```python
from build123d import *

# Parameters (mm, degrees)
SKETCH1_R           = 12.5
BOSS_EXTRUDE1_DEPTH = 5
BOSS_EXTRUDE1_TAPER = 45
FILLET2_R           = 2.5
SKETCH2_R           = 5
CUT_EXTRUDE1_DEPTH  = 3


with BuildPart() as part:
    # Sketch1 → Boss-Extrude1 (new body)
    with BuildSketch(Plane(origin=(0, 0, 0), x_dir=(1, 0, 0), z_dir=(0, 1, 0))):
        Circle(SKETCH1_R)
    extrude(amount=BOSS_EXTRUDE1_DEPTH, taper=BOSS_EXTRUDE1_TAPER)

    # Fillet2
    fillet2_edges = [part.edges().sort_by_distance(p)[0] for p in [
        (-7.5, 5, 0),
    ]]
    fillet(fillet2_edges, radius=FILLET2_R)

    # Sketch2 → Cut-Extrude1 (cut)
    with BuildSketch(Plane.XZ):
        with Locations(Location((0, 0, 0), (0, 0, 270))):
            Circle(SKETCH2_R)
    extrude(amount=-CUT_EXTRUDE1_DEPTH, mode=Mode.SUBTRACT)


solid = part.part
```
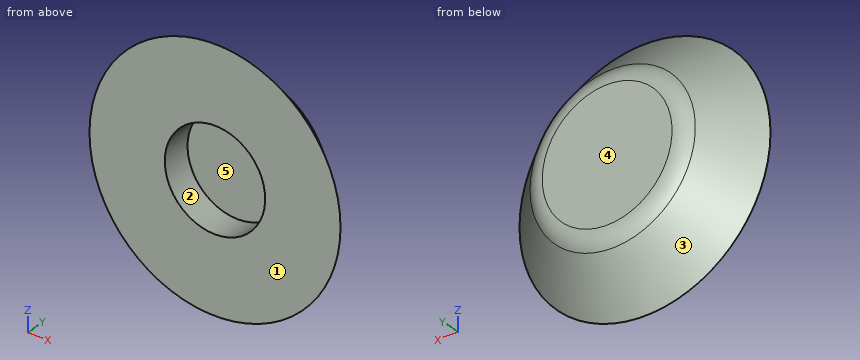
Part model, mm, in its own coordinate system. Face numbers are marked on the shaded views. A direction names the side the tool comes from. Round coordinates to 2 decimals unless told otherwise and drop trailing zeros. Loops run counter-clockwise (first coordinate to the right, second up) from the corner with the lowest first, then second, coordinate; pieces in that order, holes last.
1. Slice it at A-A (y = 1.25). Give the cut face in (x, z), and give its area (3 significant figures).
Solutions:
outline: circle Ø22.5 at (0, 0); hole circle Ø10 at (0, 0)
area: 319 mm2
2. Drill centre lines: line 1 along Y through (x, z) = (-3.5, 2.75); line 2 along X through (y, z) = (1, 3.25); line 3 along Y through (x, z) = (7.5, -8.25). Where is each one in solid material? Low to high.
Solutions:
line 1: y = 3 to 5
line 2: x = -11.03 to -3.8, 3.8 to 11.03
line 3: y = 0 to 1.35
3. Slice it at B-B (x = 0). Give the cut face in (y, z), and give its area (3 significant figures).
Solutions:
outline: (0, -12.5) - (4.27, -8.23) arc R2.5 ccw to (5, -6.46) - (5, 6.46) arc R2.5 ccw to (4.27, 8.23) - (0, 12.5) - (0, 5) - (3, 5) - (3, -5) - (0, -5) - close
area: 69.7 mm2
4. Flat gauge pins, fed straight in: pin 1 (6 mm diameter, centred on x = 0, z = 0, fed in from -Y); pin 2 (3 mm diameter, centred on y = 4.5, z = 1, fed in from +X); pin 3 (2 mm diameter, centred on x = 1.5, y = 2, fed in from +Z). Where does each tip first touch, or does it go through?
Solutions:
pin 1: stops at y = 3
pin 2: stops at x = 9.45
pin 3: stops at z = 11.41
5. Two-plate mould, pull along X, no slides. Class the marked faces 3, 4 and 5: pulls with the +X half, pulls with the -X half, needs draft (parallel to the pull), parting line crosses it, or undercut.
Solutions:
face 3: parting line crosses it
face 4: needs draft
face 5: undercut
6. 3-axis set-ups, long thin cutter, end or side, ignore diameter. For the marked faces 1 and 2: which of +Z, -Z, +X, -X, +Y, -Y reach the whole face in a straight line?
Solutions:
face 1: +Z, -Z, +X, -X, -Y
face 2: -Y
